CAD build for the part. Positions are in the model's coordinates, mm. Face numbers are marked on the shaded views. A direction names the side the tool comes from. Round coordinates to 2 decimals unless told otherwise and drop trailing zeros. Order: outer loops, then holes, each group sorted by start corner. A loop starts at its lowest first (then second) coordinate and runs counter-clockwise, first axis right, second up. Notation, with made-up numbers: M 85,77 L 117,77 A7 ccw 117,85 Z; hole C 56.25,88 d11. An arc over 180 degrees is marked long. Answer as a JSON object with one key per item and string values.
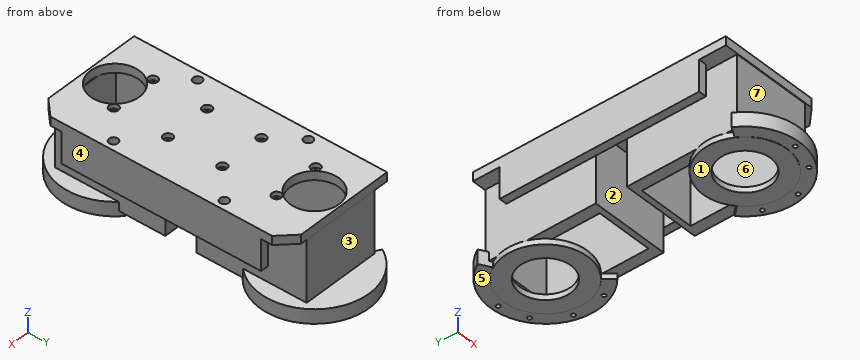
```python
from build123d import *

# Parameters (mm, degrees)
BOSS_1_DEPTH    = 4
S_BOX2_W        = 3.5
S_BOX2_H        = 90
BOSS_2_DEPTH    = 14.5
S_BOX3_W        = 3.5
S_BOX3_H        = 90
BOSS_3_DEPTH    = 14.5
S_BOX4_W        = 35.52
S_BOX4_H        = 2.5
BOSS_4_DEPTH    = 36
S_BOX5_W        = 35.52
S_BOX5_H        = 1.2
BOSS_5_DEPTH    = 36
S_BOX6_W        = 5
S_BOX6_H        = 49.72
BOSS_6_DEPTH    = 36
S_BOX7_W        = 5
S_BOX7_H        = 49.72
BOSS_7_DEPTH    = 36
S_BOX8_W        = 35.52
S_BOX8_H        = 49.72
BOSS_8_DEPTH    = 4
S_CYL9_R        = 19
BOSS_9_DEPTH    = 2.525
BOSS_10_DEPTH   = 6.4
S_BOX11_W       = 35.52
S_BOX11_H       = 1.2
BOSS_11_DEPTH   = 36
S_BOX12_W       = 35.52
S_BOX12_H       = 2.5
BOSS_12_DEPTH   = 36
S_BOX13_W       = 5
S_BOX13_H       = 49.72
BOSS_13_DEPTH   = 36
S_BOX14_W       = 5
S_BOX14_H       = 49.72
BOSS_14_DEPTH   = 36
S_BOX15_W       = 35.52
S_BOX15_H       = 49.72
BOSS_15_DEPTH   = 4
S_CYL16_R       = 19
BOSS_16_DEPTH   = 2.525
BOSS_17_DEPTH   = 6.4
S_HOLE18_R      = 11
HOLE_18_DEPTH   = 4.2
S_HOLE19_R      = 1.1
HOLE_19_DEPTH   = 4.2
S_HOLE20_R      = 2.1
HOLE_20_DEPTH   = 2.1
S_HOLE21_R      = 1.1
HOLE_21_DEPTH   = 4.2
S_HOLE22_R      = 2.1
HOLE_22_DEPTH   = 2.1
S_HOLE23_R      = 1.1
HOLE_23_DEPTH   = 4.2
S_HOLE24_R      = 2.1
HOLE_24_DEPTH   = 2.1
S_HOLE25_R      = 1.1
HOLE_25_DEPTH   = 4.2
S_HOLE26_R      = 2.1
HOLE_26_DEPTH   = 2.1
S_CUT27_W       = 25.52
S_CUT27_H       = 46.02
POCKET_27_DEPTH = 4.075
S_HOLE28_R      = 11.5
HOLE_28_DEPTH   = 2.625
S_HOLE29_R      = 0.9
HOLE_29_DEPTH   = 5.7
S_HOLE30_R      = 0.9
HOLE_30_DEPTH   = 5.7
S_HOLE31_R      = 0.9
HOLE_31_DEPTH   = 5.7
S_HOLE32_R      = 0.9
HOLE_32_DEPTH   = 5.7
S_HOLE33_R      = 11
HOLE_33_DEPTH   = 4.2
S_HOLE34_R      = 1.1
HOLE_34_DEPTH   = 4.2
S_HOLE35_R      = 2.1
HOLE_35_DEPTH   = 2.1
S_HOLE36_R      = 1.1
HOLE_36_DEPTH   = 4.2
S_HOLE37_R      = 2.1
HOLE_37_DEPTH   = 2.1
S_HOLE38_R      = 1.1
HOLE_38_DEPTH   = 4.2
S_HOLE39_R      = 2.1
HOLE_39_DEPTH   = 2.1
S_HOLE40_R      = 1.1
HOLE_40_DEPTH   = 4.2
S_HOLE41_R      = 2.1
HOLE_41_DEPTH   = 2.1
S_CUT42_W       = 25.52
S_CUT42_H       = 46.02
POCKET_42_DEPTH = 4.075
S_HOLE43_R      = 11.5
HOLE_43_DEPTH   = 2.625
S_HOLE44_R      = 0.9
HOLE_44_DEPTH   = 5.7
S_HOLE45_R      = 0.9
HOLE_45_DEPTH   = 5.7
S_HOLE46_R      = 0.9
HOLE_46_DEPTH   = 5.7
S_HOLE47_R      = 0.9
HOLE_47_DEPTH   = 5.7
S_HOLE48_R      = 2
HOLE_48_DEPTH   = 4.2
S_HOLE49_R      = 2
HOLE_49_DEPTH   = 4.2
S_HOLE50_R      = 2
HOLE_50_DEPTH   = 4.2
S_HOLE51_R      = 2
HOLE_51_DEPTH   = 4.2


with BuildPart() as part:
    # S_prism1 → Boss_1 (new body)
    with BuildSketch(Plane.XY.offset(64.625)):
        Polygon((28, -50), (28, 50), (21, 57), (-24, 57), (-24, -57), (21, -57), align=None)
    extrude(amount=BOSS_1_DEPTH)

    # S_box2 → Boss_2 (add)
    with BuildSketch(Plane.XY.offset(50.625)):
        with Locations((26.25, 0)):
            Rectangle(S_BOX2_W, S_BOX2_H)
    extrude(amount=BOSS_2_DEPTH)

    # S_box3 → Boss_3 (add)
    with BuildSketch(Plane.XY.offset(50.625)):
        with Locations((-22.25, 0)):
            Rectangle(S_BOX3_W, S_BOX3_H)
    extrude(amount=BOSS_3_DEPTH)

    # S_box4 → Boss_4 (add)
    with BuildSketch(Plane.XY.offset(32.625)):
        with Locations((0, 8.24)):
            Rectangle(S_BOX4_W, S_BOX4_H)
    extrude(amount=BOSS_4_DEPTH)

    # S_box5 → Boss_5 (add)
    with BuildSketch(Plane.XY.offset(32.625)):
        with Locations((0, 56.11)):
            Rectangle(S_BOX5_W, S_BOX5_H)
    extrude(amount=BOSS_5_DEPTH)

    # S_box6 → Boss_6 (add)
    with BuildSketch(Plane.XY.offset(32.625)):
        with Locations((-15.26, 31.85)):
            Rectangle(S_BOX6_W, S_BOX6_H)
    extrude(amount=BOSS_6_DEPTH)

    # S_box7 → Boss_7 (add)
    with BuildSketch(Plane.XY.offset(32.625)):
        with Locations((15.26, 31.85)):
            Rectangle(S_BOX7_W, S_BOX7_H)
    extrude(amount=BOSS_7_DEPTH)

    # S_box8 → Boss_8 (add)
    with BuildSketch(Plane.XY.offset(64.625)):
        with Locations((0, 31.85)):
            Rectangle(S_BOX8_W, S_BOX8_H)
    extrude(amount=BOSS_8_DEPTH)

    # S_cyl9 → Boss_9 (add)
    with BuildSketch(Plane.XY.offset(30.1)):
        with Locations(Location((0, 45, 0), (0, 0, 200.814328514))):
            Circle(S_CYL9_R)
    extrude(amount=BOSS_9_DEPTH)

    # S_prism10 → Boss_10 (add)
    with BuildSketch(Plane.XY.offset(30.2)):
        with BuildLine():
            Line((-21.304224933, 57.3), (-9.526279442, 50.5))
            ThreePointArc((-9.526279442, 50.5), (6.996860423, 53.487870417), (7.216649319, 36.698194618))
            Line((7.216649319, 36.698194618), (16.139052113, 26.434144327))
            ThreePointArc((16.139052113, 26.434144327), (15.647524219, 63.981964751), (-21.304224933, 57.3))
        make_face()
    extrude(amount=BOSS_10_DEPTH)

    # S_box11 → Boss_11 (add)
    with BuildSketch(Plane.XY.offset(32.625)):
        with Locations((0, -56.11)):
            Rectangle(S_BOX11_W, S_BOX11_H)
    extrude(amount=BOSS_11_DEPTH)

    # S_box12 → Boss_12 (add)
    with BuildSketch(Plane.XY.offset(32.625)):
        with Locations((0, -8.24)):
            Rectangle(S_BOX12_W, S_BOX12_H)
    extrude(amount=BOSS_12_DEPTH)

    # S_box13 → Boss_13 (add)
    with BuildSketch(Plane.XY.offset(32.625)):
        with Locations((-15.26, -31.85)):
            Rectangle(S_BOX13_W, S_BOX13_H)
    extrude(amount=BOSS_13_DEPTH)

    # S_box14 → Boss_14 (add)
    with BuildSketch(Plane.XY.offset(32.625)):
        with Locations((15.26, -31.85)):
            Rectangle(S_BOX14_W, S_BOX14_H)
    extrude(amount=BOSS_14_DEPTH)

    # S_box15 → Boss_15 (add)
    with BuildSketch(Plane.XY.offset(64.625)):
        with Locations((0, -31.85)):
            Rectangle(S_BOX15_W, S_BOX15_H)
    extrude(amount=BOSS_15_DEPTH)

    # S_cyl16 → Boss_16 (add)
    with BuildSketch(Plane.XY.offset(30.1)):
        with Locations(Location((0, -45, 0), (0, 0, 200.814328514))):
            Circle(S_CYL16_R)
    extrude(amount=BOSS_16_DEPTH)

    # S_prism17 → Boss_17 (add)
    with BuildSketch(Plane.XY.offset(30.2)):
        with BuildLine():
            Line((16.139052113, -26.434144327), (7.216649319, -36.698194618))
            ThreePointArc((7.216649319, -36.698194618), (6.996860423, -53.487870417), (-9.526279442, -50.5))
            Line((-9.526279442, -50.5), (-21.304224933, -57.3))
            ThreePointArc((-21.304224933, -57.3), (15.647524219, -63.981964751), (16.139052113, -26.434144327))
        make_face()
    extrude(amount=BOSS_17_DEPTH)

    # S_hole18 → Hole_18 (cut)
    with BuildSketch(Plane.XY.offset(64.525)):
        with Locations(Location((0, 45, 0), (0, 0, 107.165830165))):
            Circle(S_HOLE18_R)
    extrude(amount=HOLE_18_DEPTH, mode=Mode.SUBTRACT)

    # S_hole19 → Hole_19 (cut)
    with BuildSketch(Plane.XY.offset(64.525)):
        with Locations((-10.25, 36.7)):
            Circle(S_HOLE19_R)
    extrude(amount=HOLE_19_DEPTH, mode=Mode.SUBTRACT)

    # S_hole20 → Hole_20 (cut)
    with BuildSketch(Plane.XY.offset(66.625)):
        with Locations((-10.25, 36.7)):
            Circle(S_HOLE20_R)
    extrude(amount=HOLE_20_DEPTH, mode=Mode.SUBTRACT)

    # S_hole21 → Hole_21 (cut)
    with BuildSketch(Plane.XY.offset(64.525)):
        with Locations((10.25, 36.7)):
            Circle(S_HOLE21_R)
    extrude(amount=HOLE_21_DEPTH, mode=Mode.SUBTRACT)

    # S_hole22 → Hole_22 (cut)
    with BuildSketch(Plane.XY.offset(66.625)):
        with Locations((10.25, 36.7)):
            Circle(S_HOLE22_R)
    extrude(amount=HOLE_22_DEPTH, mode=Mode.SUBTRACT)

    # S_hole23 → Hole_23 (cut)
    with BuildSketch(Plane.XY.offset(64.525)):
        with Locations((-10.25, 12.25)):
            Circle(S_HOLE23_R)
    extrude(amount=HOLE_23_DEPTH, mode=Mode.SUBTRACT)

    # S_hole24 → Hole_24 (cut)
    with BuildSketch(Plane.XY.offset(66.625)):
        with Locations((-10.25, 12.25)):
            Circle(S_HOLE24_R)
    extrude(amount=HOLE_24_DEPTH, mode=Mode.SUBTRACT)

    # S_hole25 → Hole_25 (cut)
    with BuildSketch(Plane.XY.offset(64.525)):
        with Locations((10.25, 12.25)):
            Circle(S_HOLE25_R)
    extrude(amount=HOLE_25_DEPTH, mode=Mode.SUBTRACT)

    # S_hole26 → Hole_26 (cut)
    with BuildSketch(Plane.XY.offset(66.625)):
        with Locations((10.25, 12.25)):
            Circle(S_HOLE26_R)
    extrude(amount=HOLE_26_DEPTH, mode=Mode.SUBTRACT)

    # S_cut27 → Pocket_27 (cut)
    with BuildSketch(Plane.XY.offset(32.625)):
        with Locations((0, 32.5)):
            Rectangle(S_CUT27_W, S_CUT27_H)
    extrude(amount=POCKET_27_DEPTH, mode=Mode.SUBTRACT)

    # S_hole28 → Hole_28 (cut)
    with BuildSketch(Plane.XY.offset(30.1)):
        with Locations(Location((0, 45, 0), (0, 0, 113.948166611))):
            Circle(S_HOLE28_R)
    extrude(amount=HOLE_28_DEPTH, mode=Mode.SUBTRACT)

    # S_hole29 → Hole_29 (cut)
    with BuildSketch(Plane.XY.offset(30.1)):
        with Locations((19.938771315, 35.702398242)):
            Circle(S_HOLE29_R)
    extrude(amount=HOLE_29_DEPTH, mode=Mode.SUBTRACT)

    # S_hole30 → Hole_30 (cut)
    with BuildSketch(Plane.XY.offset(30.1)):
        with Locations((21.250368178, 50.694018992)):
            Circle(S_HOLE30_R)
    extrude(amount=HOLE_30_DEPTH, mode=Mode.SUBTRACT)

    # S_hole31 → Hole_31 (cut)
    with BuildSketch(Plane.XY.offset(30.1)):
        with Locations((12.6186816, 63.021344974)):
            Circle(S_HOLE31_R)
    extrude(amount=HOLE_31_DEPTH, mode=Mode.SUBTRACT)

    # S_hole32 → Hole_32 (cut)
    with BuildSketch(Plane.XY.offset(30.1)):
        with Locations((0.767788927, 66.986598194)):
            Circle(S_HOLE32_R)
    extrude(amount=HOLE_32_DEPTH, mode=Mode.SUBTRACT)

    # S_hole33 → Hole_33 (cut)
    with BuildSketch(Plane.XY.offset(64.525)):
        with Locations(Location((0, -45, 0), (0, 0, 252.834169835))):
            Circle(S_HOLE33_R)
    extrude(amount=HOLE_33_DEPTH, mode=Mode.SUBTRACT)

    # S_hole34 → Hole_34 (cut)
    with BuildSketch(Plane.XY.offset(64.525)):
        with Locations((-10.25, -36.7)):
            Circle(S_HOLE34_R)
    extrude(amount=HOLE_34_DEPTH, mode=Mode.SUBTRACT)

    # S_hole35 → Hole_35 (cut)
    with BuildSketch(Plane.XY.offset(66.625)):
        with Locations((-10.25, -36.7)):
            Circle(S_HOLE35_R)
    extrude(amount=HOLE_35_DEPTH, mode=Mode.SUBTRACT)

    # S_hole36 → Hole_36 (cut)
    with BuildSketch(Plane.XY.offset(64.525)):
        with Locations((10.25, -36.7)):
            Circle(S_HOLE36_R)
    extrude(amount=HOLE_36_DEPTH, mode=Mode.SUBTRACT)

    # S_hole37 → Hole_37 (cut)
    with BuildSketch(Plane.XY.offset(66.625)):
        with Locations((10.25, -36.7)):
            Circle(S_HOLE37_R)
    extrude(amount=HOLE_37_DEPTH, mode=Mode.SUBTRACT)

    # S_hole38 → Hole_38 (cut)
    with BuildSketch(Plane.XY.offset(64.525)):
        with Locations((-10.25, -12.25)):
            Circle(S_HOLE38_R)
    extrude(amount=HOLE_38_DEPTH, mode=Mode.SUBTRACT)

    # S_hole39 → Hole_39 (cut)
    with BuildSketch(Plane.XY.offset(66.625)):
        with Locations((-10.25, -12.25)):
            Circle(S_HOLE39_R)
    extrude(amount=HOLE_39_DEPTH, mode=Mode.SUBTRACT)

    # S_hole40 → Hole_40 (cut)
    with BuildSketch(Plane.XY.offset(64.525)):
        with Locations((10.25, -12.25)):
            Circle(S_HOLE40_R)
    extrude(amount=HOLE_40_DEPTH, mode=Mode.SUBTRACT)

    # S_hole41 → Hole_41 (cut)
    with BuildSketch(Plane.XY.offset(66.625)):
        with Locations((10.25, -12.25)):
            Circle(S_HOLE41_R)
    extrude(amount=HOLE_41_DEPTH, mode=Mode.SUBTRACT)

    # S_cut42 → Pocket_42 (cut)
    with BuildSketch(Plane.XY.offset(32.625)):
        with Locations((0, -32.5)):
            Rectangle(S_CUT42_W, S_CUT42_H)
    extrude(amount=POCKET_42_DEPTH, mode=Mode.SUBTRACT)

    # S_hole43 → Hole_43 (cut)
    with BuildSketch(Plane.XY.offset(30.1)):
        with Locations(Location((0, -45, 0), (0, 0, 246.051833389))):
            Circle(S_HOLE43_R)
    extrude(amount=HOLE_43_DEPTH, mode=Mode.SUBTRACT)

    # S_hole44 → Hole_44 (cut)
    with BuildSketch(Plane.XY.offset(30.1)):
        with Locations((19.938771315, -35.702398242)):
            Circle(S_HOLE44_R)
    extrude(amount=HOLE_44_DEPTH, mode=Mode.SUBTRACT)

    # S_hole45 → Hole_45 (cut)
    with BuildSketch(Plane.XY.offset(30.1)):
        with Locations((21.250368178, -50.694018992)):
            Circle(S_HOLE45_R)
    extrude(amount=HOLE_45_DEPTH, mode=Mode.SUBTRACT)

    # S_hole46 → Hole_46 (cut)
    with BuildSketch(Plane.XY.offset(30.1)):
        with Locations((12.6186816, -63.021344974)):
            Circle(S_HOLE46_R)
    extrude(amount=HOLE_46_DEPTH, mode=Mode.SUBTRACT)

    # S_hole47 → Hole_47 (cut)
    with BuildSketch(Plane.XY.offset(30.1)):
        with Locations((0.767788927, -66.986598194)):
            Circle(S_HOLE47_R)
    extrude(amount=HOLE_47_DEPTH, mode=Mode.SUBTRACT)

    # S_hole48 → Hole_48 (cut)
    with BuildSketch(Plane.XY.offset(64.525)):
        with Locations(Location((-20, -25, 0), (0, 0, 255.522487814))):
            Circle(S_HOLE48_R)
    extrude(amount=HOLE_48_DEPTH, mode=Mode.SUBTRACT)

    # S_hole49 → Hole_49 (cut)
    with BuildSketch(Plane.XY.offset(64.525)):
        with Locations(Location((-20, 25, 0), (0, 0, 255.522487814))):
            Circle(S_HOLE49_R)
    extrude(amount=HOLE_49_DEPTH, mode=Mode.SUBTRACT)

    # S_hole50 → Hole_50 (cut)
    with BuildSketch(Plane.XY.offset(64.525)):
        with Locations(Location((24, -25, 0), (0, 0, 284.477512186))):
            Circle(S_HOLE50_R)
    extrude(amount=HOLE_50_DEPTH, mode=Mode.SUBTRACT)

    # S_hole51 → Hole_51 (cut)
    with BuildSketch(Plane.XY.offset(64.525)):
        with Locations(Location((24, 25, 0), (0, 0, 284.477512186))):
            Circle(S_HOLE51_R)
    extrude(amount=HOLE_51_DEPTH, mode=Mode.SUBTRACT)


solid = part.part
```
Item 1: 3-axis set-ups, long thin cutter, end or side, ignore diameter. For the marked faces 4, 5, 6 and 7: which of +Z, -Z, +X, -X, +Y, -Y reach the whole face in a straight line?
Worked answers:
{"face 4": "+Z, -Z, +X, +Y, -Y", "face 5": "-Z", "face 6": "none", "face 7": "+X, -X, -Y"}
Item 2: Saw through at A-A on z = 38. List the corners of the cut face in (x, y).
Worked answers:
{"outline": "M -17.76,-56.71 L 17.76,-56.71 L 17.76,-6.99 L -17.76,-6.99 Z; M -17.76,6.99 L 17.76,6.99 L 17.76,56.71 L -17.76,56.71 Z; hole M -12.76,-55.51 L 12.76,-55.51 L 12.76,-9.49 L -12.76,-9.49 Z; hole M -12.76,9.49 L 12.76,9.49 L 12.76,55.51 L -12.76,55.51 Z"}
Item 3: Saw through at B-B on y = -16. List the corners of the cut face in (x, z) (3 decimals).
Worked answers:
{"outline": "M -24,50.625 L -20.5,50.625 L -20.5,64.625 L -17.76,64.625 L -17.76,32.625 L -12.76,32.625 L -12.76,64.625 L 12.76,64.625 L 12.76,32.625 L 17.76,32.625 L 17.76,64.625 L 24.5,64.625 L 24.5,50.625 L 28,50.625 L 28,68.625 L -24,68.625 Z"}
Item 4: Wall check: line 1 along X through (y, z) = (-25, 67.3); line 2 along Y through (x, z) = (0, 52); line 3 along X through (y, z) = (14, 53.5). Give the ranges that are in metal, low to high. Write a range as [from, to].
Worked answers:
{"line 1": "x = [-24, -22], [-18, 22], [26, 28]", "line 2": "y = [-56.71, -55.51], [-9.49, -6.99], [6.99, 9.49], [55.51, 56.71]", "line 3": "x = [-24, -20.5], [-17.76, -12.76], [12.76, 17.76], [24.5, 28]"}
Item 5: Drop flat-ended pins along their axis: pin 1 Ø20.5 at (x, y) = (-3.5, 25.5) entering from -Z; pin 2 Ø5 at (x, z) = (-3.5, 36.5) entering from +Y; pin 3 Ø10 at (x, z) = (-7, 45.5) entering from -Y; pin 4 Ø6 at (x, z) = (-13, 47) entering from +Y. Give the stop position or say it passes through.
Worked answers:
{"pin 1": "stops at z = 30.1", "pin 2": "stops at y = 69.58", "pin 3": "stops at y = -56.71", "pin 4": "stops at y = 56.71"}
Item 6: Two-plate mould, pull along Z, no slides. Class the marked faces 1, 2 and 3: released by +Z, released by -Z, zero draft, split by the parting line, or undercut.
Worked answers:
{"face 1": "released by -Z", "face 2": "zero draft", "face 3": "undercut"}
Item 7: Saw through at C-C on y = -59. List the corners of the cut face in (x, z), and give its area (3 significant figures).
Worked answers:
{"outline": "M -20.23,30.2 L -12.85,30.2 L -12.85,30.1 L 12.85,30.1 L 12.85,30.2 L 20.23,30.2 L 20.23,36.6 L -20.23,36.6 Z", "area": "261 mm2"}
